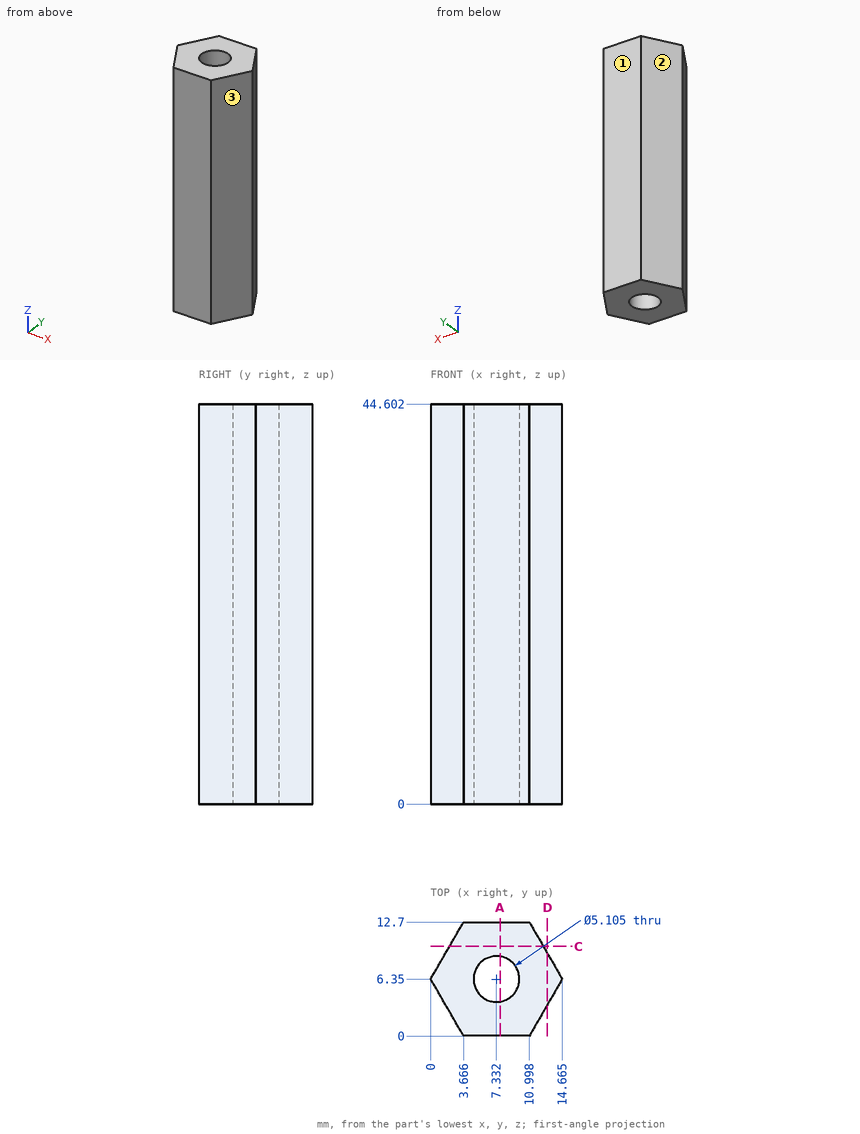
Part print with two shaded views. Sizes in mm from the minimum x, y, z corner. Round coordinates to 2 decimals unless told otherwise and drop trailing zeros. Write each loop counter-clockwise with the first axis right and the second up, starting at its lowest first coordinate (ties: lowest second). Pieces come first, ordered by that corner, then holes. Notation, with made-up numbers: (-4, 54.25) -> (25, 54.25) arc R31 ccw to (25, 83.25) -> close; hole circle Ø5 at (71, 48). An arc over 180 degrees is marked (long way). Use one line per item in the form item = value.
Q1. Two-plate mould, pull along X, no slides. Class the marked faces 1, 2 and 3: released by +X, released by -X, zero draft, split by the parting line, or undercut.
Conclusion:
face_1 = zero draft
face_2 = released by -X
face_3 = released by +X
Q2. Drop flat-ended pins along their axis: P1, Ø1, axis at x = 12.5, z = 15.5, coming from the -Y side (1 decimal); P2, Ø3, axis at x = 7.33, y = 6.35, coming from the -Z side; P3, Ø2, axis at y = 4.5, z = 22, coming from the -X side; P4, Ø4, axis at y = 5, z = 5, coming from the +X side (1 decimal). Give the stop position or say it passes through.
Conclusion:
P1 = 1.7
P2 = through
P3 = 0.49
P4 = 14.7
Q3. Band-saw the part on C-C, the plane y = 10. Write the cut outline in (x, z).
Conclusion:
outline = (2.11, 0) -> (12.56, 0) -> (12.56, 44.6) -> (2.11, 44.6) -> close
Q4. Band-saw the part on D-D, the plane x = 13. Write the cut outline in (y, z).
Conclusion:
outline = (3.47, 0) -> (9.23, 0) -> (9.23, 44.6) -> (3.47, 44.6) -> close
Q5. Band-saw the part on A-A, the plane x = 7.75. Write the cut outline in (y, z).
Conclusion:
outline = (0, 0) -> (3.83, 0) -> (3.83, 44.6) -> (0, 44.6) -> close; (8.87, 0) -> (12.7, 0) -> (12.7, 44.6) -> (8.87, 44.6) -> close
Q6. Drill centre lines: L1, parallel to X at y = 4, z = 9 (1 decimal); L2, parallel to X at y = 6, z = 3 (1 decimal); L3, parallel to Y at x = 6, z = 9. Where is each one in solid material? Low to high.
Conclusion:
L1 = 1.4 to 6.3, 8.3 to 13.3
L2 = 0.2 to 4.8, 9.9 to 14.5
L3 = 0 to 4.17, 8.53 to 12.7
